from build123d import *

# Parameters (mm, degrees)
SKETCH1_R           = 3.1
BOSS_EXTRUDE1_DEPTH = 3
SKETCH2_W           = 3
SKETCH2_H           = 20
BOSS_EXTRUDE2_DEPTH = 10
FILLET1_R           = 10
CUT_EXTRUDE1_DEPTH  = 60.439044407
FILLET2_R           = 1


with BuildPart() as part:
    # Sketch1 → Boss-Extrude1 (new body)
    with BuildSketch(Plane.XY):
        with BuildLine():
            Line((10, 0), (45, 0))
            Line((45, 0), (45, 30))
            ThreePointArc((45, 30), (42.071067812, 37.071067812), (35, 40))
            Line((35, 40), (10, 40))
            ThreePointArc((10, 40), (2.928932188, 37.071067812), (0, 30))
            Line((0, 30), (0, 10))
            ThreePointArc((0, 10), (2.928932188, 2.928932188), (10, 0))
        make_face()
        with Locations((23, 30)):
            Circle(SKETCH1_R, mode=Mode.SUBTRACT)
        with Locations((23, 10)):
            Circle(SKETCH1_R, mode=Mode.SUBTRACT)
    extrude(amount=BOSS_EXTRUDE1_DEPTH)

    # Sketch2 → Boss-Extrude2 (add)
    with BuildSketch(Plane.XY.offset(3)):
        with Locations((43.5, 10)):
            Rectangle(SKETCH2_W, SKETCH2_H)
    extrude(amount=BOSS_EXTRUDE2_DEPTH)

    # Fillet1
    fillet1_edges = [part.edges().sort_by_distance(p)[0] for p in [
        (43.5, 0, 13),
        (43.5, 20, 13),
    ]]
    fillet(fillet1_edges, radius=FILLET1_R - 0.0001)  # a hair under: the kernel refuses the full size

    # Sketch3 → Cut-Extrude1 (cut, through all)
    with BuildSketch(Plane.ZY.offset(-42)):
        with BuildLine():
            Line((3, 17), (3, 3))
            ThreePointArc((3, 3), (10, 10), (3, 17))
        make_face()
    extrude(amount=-CUT_EXTRUDE1_DEPTH, mode=Mode.SUBTRACT)

    # Fillet2
    fillet2_edges = [part.edges().sort_by_distance(p)[0] for p in [
        (45, 0, 1.50005),
        (45, 17.071097101, 10.071097101),
        (45, 2.928902899, 10.071097101),
        (42, 17.071097101, 10.071097101),
        (42, 2.928902899, 10.071097101),
        (45, 10, 10),
        (42, 10, 10),
    ]]
    fillet(fillet2_edges, radius=FILLET2_R)


solid = part.part
CAD build for the part. Positions are in the model's coordinates, mm. A direction names the side the tool comes from. Round coordinates to 2 decimals unless told otherwise and drop trailing zeros. Order: outer loops, then holes, each group sorted by start corner. A loop starts at its lowest first (then second) coordinate and runs counter-clockwise, first axis right, second up. Notation, with made-up numbers: (-17.75, -27.75) -> (28.25, -27.75) arc R22 ccw to (28.25, -1.75) -> close; hole circle Ø9 at (78, 69). An arc over 180 degrees is marked (long way). Write each question's results on one line, items separated by ' | '.
1. Cut at C-C (y = 32.5). Give the cut face in (x, z).
Findings below:
outline: (0.32, 0) -> (21.17, 0) -> (21.17, 3) -> (0.32, 3) -> close; (24.83, 0) -> (44.68, 0) -> (44.68, 3) -> (24.83, 3) -> close
2. Flat gauge pins, fed straight in: P1, Ø6, axis at x = 16.5, y = 11.5, coming from the +Z side; P2, Ø2, axis at y = 19, z = 5, coming from the -X side; P3, Ø4, axis at x = 23, z = 4, coming from the +Y side. Where does each tip first touch, or does it go through?
Findings below:
P1: stops at z = 3 | P2: stops at x = 42 | P3: stops at y = 40
3. Cut at A-A (z = 1.5). Give the cut face in (x, y), plus the area to 3 significant figures.
Findings below:
outline: (0, 10) arc R10 ccw to (10, 0) -> (44, 0) arc R1 ccw to (45, 1) -> (45, 30) arc R10 ccw to (35, 40) -> (10, 40) arc R10 ccw to (0, 30) -> close; hole circle Ø6.2 at (23, 10); hole circle Ø6.2 at (23, 30) | area: 1,680 mm²
4. 3-axis set-ups, long thin cutter, end or side, ignore diameter. For faces 1 (the face through (45, 13, 2)), 2 (the face through (42, 9.96, 11.15)), 3 (the face through (43.49, 9.85, 10)): which of +Z, -Z, +X, -X, +Y, -Y reach the whole face in a straight line?
Findings below:
face 1: +Z, -Z, +X, +Y, -Y | face 2: +Z, -X, +Y, -Y | face 3: +X, -X
5. Cut at D-D (x = 29). Give the cut face in (y, z).
Findings below:
outline: (0, 0) -> (40, 0) -> (40, 3) -> (0, 3) -> close
6. Wall check: line 1 along Y through (x, z) = (23, 1.6); line 2 along Z through (x, y) = (3, 25); line 3 along X through (y, z) = (8.5, 10.75). Give the ranges that are in metal, low to high. Write a range as [from, to].
Findings below:
line 1: y = [0, 6.9], [13.1, 26.9], [33.1, 40] | line 2: z = [0, 3] | line 3: x = [42.01, 44.99]
7. Cut at B-B (x = 23). Give the cut face in (y, z), plus the area to 3 significant figures.
Findings below:
outline: (0, 0) -> (6.9, 0) -> (6.9, 3) -> (0, 3) -> close; (13.1, 0) -> (26.9, 0) -> (26.9, 3) -> (13.1, 3) -> close; (33.1, 0) -> (40, 0) -> (40, 3) -> (33.1, 3) -> close | area: 82.8 mm²
8. Pull direction Y, two halves, no side cores. Call faces 4 (the face through (2.85, 3.01, 1.48)), 5 (the face through (22, 20, 0)), 6 (the face through (20.72, 32.1, 1.48)), 7 (the face through (23, 40, 1)): pulls with the +Y half, pulls with the -Y half, needs draft (parallel to the pull), parting line crosses it, or undercut.
Findings below:
face 4: pulls with the -Y half | face 5: needs draft | face 6: undercut | face 7: pulls with the +Y half
